```python
from build123d import *

# Parameters (mm, degrees)
F0_R     = 2.55
F1_DEPTH = 36
F2_W     = 30
F2_H     = 13
F3_DEPTH = 8
F4_R     = 10
F5_R     = 5


with BuildPart() as f1:
    # F0 (on Top) → F1 (new body)
    with BuildSketch(Plane.XY):
        with BuildLine():
            ThreePointArc((4, 30.065), (0, 34.065), (-4, 30.065))
            Line((-4, 30.065), (-4, -30.065))
            ThreePointArc((-4, -30.065), (0, -34.065), (4, -30.065))
            Line((4, -30.065), (4, 30.065))
        make_face()
        with Locations((0, -30.065)):
            Circle(F0_R, mode=Mode.SUBTRACT)
        with Locations((0, 30.065)):
            Circle(F0_R, mode=Mode.SUBTRACT)
    extrude(amount=F1_DEPTH)

    # F2 (on face) → F3 (cut, through all)
    with BuildSketch(Plane(origin=(-4, 0, 0), x_dir=(0, -1, 0), z_dir=(-1, 0, 0))):
        with Locations((0, 29.5)):
            Rectangle(F2_W, F2_H)
        with Locations((0, 6.5)):
            Rectangle(F2_W, F2_H)
    extrude(amount=-F3_DEPTH, mode=Mode.SUBTRACT)

    # F4
    f4_edges = [f1.edges().sort_by_distance(p)[0] for p in [
        (0, 15, 36),
        (0, 15, 0),
        (0, -15, 0),
        (0, -15, 36),
    ]]
    fillet(f4_edges, radius=F4_R)

    # F5
    f5_edges = [f1.edges().sort_by_distance(p)[0] for p in [
        (0, 15, 23),
        (0, -15, 23),
        (0, -15, 13),
        (0, 15, 13),
    ]]
    fillet(f5_edges, radius=F5_R)


solid = f1.part
```
Model file for the job. Use its own axes, mm. A direction names the side the tool comes from. Round coordinates to 2 decimals unless told otherwise and drop trailing zeros. Loops run counter-clockwise (first coordinate to the right, second up) from the corner with the lowest first, then second, coordinate; pieces in that order, holes last. Notation, with made-up numbers: M -3,16.25 L 41,16.25 A28 ccw 41,45.25 Z; hole C 52,24.5 d5. An arc over 180 degrees is marked long. Put each result on its own line as item: value. Start each with the question number.
Item 1: Drop flat-ended pins along their axis: P1, Ø4, axis at x = 1.5, y = 9, coming from the -Z side; P2, Ø4, axis at x = -1, y = 4.5, coming from the +Z side; P3, Ø3, axis at x = -2.5, z = 25, coming from the -Y side. Give the stop position or say it passes through.
Item 2: Mould opens along Y. For faces 1 (the face through (0.06, -18.34, 33.46)), 2 (the face through (0.088, 34.064, 17.748)), 3 (the face through (2, 28, 0)) say: released by +Y, released by -Y, zero draft, split by the parting line, or undercut.
Item 3: Cut at C-C (x = 0). Give the number of separate pieces and of enclosed holes in the cut face, then the cut area to 3 significant figures.
Item 4: Cut at A-A (z = 33). List the corners of the cut face in (x, y) (3 decimals), then the cut area to 3 significant figures.
Item 5: Cut at B-B (z = 21.5). List the corners of the cut face in (x, y) (3 decimals).
Item 6: Drill centre lines: line 1 along Y through (x, z) = (0, 17) (3 decimals); line 2 along Y through (x, z) = (1, 15); line 3 along Y through (x, z) = (0, 8) (3 decimals). Where is each one in solid material? Low to high.
Item 7: Cut at D-D (y = -6). List the corners of the cut face in (x, z).
Item 8: 3-axis set-ups, long thin cutter, end or side, ignore diameter. For faces 4 (the face through (0, 0, 13)), 5 (the face through (-4, 0, 18)), 6 (the face through (0.1, 18.5, 33.6)): which of +Z, -Z, +X, -X, +Y, -Y reach the whole face in a straight line?
Answer block:
1. P1: z = 12.92
1. P2: z = 23
1. P3: y = -33.94
2. face 1: undercut
2. face 2: released by +Y
2. face 3: zero draft
3. separate pieces: 3
3. enclosed holes: 0
3. area: 1,240 mm2
4. outline: M -4,-30.065 A4 ccw 4,-30.065 L 4,-17.859 L -4,-17.859 Z; M -4,17.859 L 4,17.859 L 4,30.065 A4 ccw -4,30.065 Z; hole C 0,-30.065 d5.1; hole C 0,30.065 d5.1
4. area: 205 mm2
5. outline: M -4,-30.065 A4 ccw 4,-30.065 L 4,30.065 A4 ccw -4,30.065 Z; hole C 0,-30.065 d5.1; hole C 0,30.065 d5.1
6. line 1: -34.065 to -32.615, -27.515 to 27.515, 32.615 to 34.065
6. line 2: -33.94 to -32.41, -27.72 to 27.72, 32.41 to 33.94
6. line 3: -34.065 to -32.615, -27.515 to -15.202, 15.202 to 27.515, 32.615 to 34.065
7. outline: M -4,13 L 4,13 L 4,23 L -4,23 Z
8. face 4: -Z, +X, -X
8. face 5: +Z, -Z, -X, +Y, -Y
8. face 6: +Z, +X, -X
